CAD build for the part. Positions are in the model's coordinates, mm. Round coordinates to 2 decimals unless told otherwise and drop trailing zeros. Order: outer loops, then holes, each group sorted by start corner. A loop starts at its lowest first (then second) coordinate and runs counter-clockwise, first axis right, second up. Notation, with made-up numbers: M 49,-36 L 108,-36 A8 cw 108,-22 Z; hole C -10,-36.75 d1. An arc over 180 degrees is marked long. Answer as a JSON object with one key per item and string values.
```python
from build123d import *

# Parameters (mm, degrees)
F0_R     = 1.5875
F1_DEPTH = 3.048


# Not quite as in the source:
# - a feature names something its author has since deleted; it is built from what else it names


with BuildPart() as f1:
    # F0 (on Front) → F1 (new body)
    with BuildSketch(Plane.XZ):
        with BuildLine():
            Line((0, 3.0934604908), (0, 0))
            Line((0, 0), (0, -9.6065395092))
            ThreePointArc((0, -9.6065395092), (11.1386616751, -5.0428542466), (15.8731222627, 6.024299409))
            ThreePointArc((15.8731222627, 6.024299409), (15.8745305587, 6.1463763397), (15.875, 6.2684604908))
            ThreePointArc((15.875, 6.2684604908), (15.8438414904, 7.2625992274), (15.7504882737, 8.2528354908))
            ThreePointArc((15.7504882737, 8.2528354908), (10.5003255158, 18.1747104908), (0, 22.1434604908))
            Line((0, 22.1434604908), (0, 9.4434604908))
            ThreePointArc((0, 9.4434604908), (2.2450640303, 8.513524521), (3.175, 6.2684604908))
            ThreePointArc((3.175, 6.2684604908), (2.2450640303, 4.0233964605), (0, 3.0934604908))
        make_face()
        with BuildLine():
            Line((0, -9.6065395092), (0, 0))
            Line((0, 0), (0, 3.0934604908))
            ThreePointArc((0, 3.0934604908), (-3.175, 6.2684604908), (0, 9.4434604908))
            Line((0, 9.4434604908), (0, 22.1434604908))
            ThreePointArc((0, 22.1434604908), (-10.5003255158, 18.1747104908), (-15.7504882737, 8.2528354908))
            ThreePointArc((-15.7504882737, 8.2528354908), (-15.8510182356, 7.1407252981), (-15.8731222627, 6.024299409))
            ThreePointArc((-15.8731222627, 6.024299409), (-11.1386616751, -5.0428542466), (0, -9.6065395092))
        make_face()
        with BuildLine():
            ThreePointArc((15.8731222627, 6.024299409), (11.1386616751, -5.0428542466), (0, -9.6065395092))
            Line((0, -9.6065395092), (0, -42.3331838364))
            ThreePointArc((0, -42.3331838364), (10.5347283248, -46.6968111845), (14.8983556728, -57.2315395092))
            Line((14.8983556728, -57.2315395092), (36.5125, -57.2315395092))
            ThreePointArc((36.5125, -57.2315395092), (39.2955109449, -51.1953860295), (45.6930099416, -49.3919711196))
            Line((45.6930099416, -49.3919711196), (21.9056452954, -45.6203437456))
            ThreePointArc((21.9056452954, -45.6203437456), (17.0653083108, -42.8843212703), (15.2013844237, -37.6459561768))
            Line((15.2013844237, -37.6459561768), (15.8731222627, 6.024299409))
        make_face()
        with BuildLine():
            Line((0, -42.3331838364), (0, -9.6065395092))
            ThreePointArc((0, -9.6065395092), (-11.1386616751, -5.0428542466), (-15.8731222627, 6.024299409))
            Line((-15.8731222627, 6.024299409), (-14.8965934556, -57.4606795809))
            ThreePointArc((-14.8965934556, -57.4606795809), (-10.6154324462, -46.778138353), (0, -42.3331838364))
        make_face()
        with BuildLine():
            ThreePointArc((14.8983556728, -57.2315395092), (10.5347283248, -46.6968111845), (0, -42.3331838364))
            Line((0, -42.3331838364), (0, -54.0565395092))
            ThreePointArc((0, -54.0565395092), (2.2450640303, -54.986475479), (3.175, -57.2315395092))
            Line((3.175, -57.2315395092), (14.8983556728, -57.2315395092))
        make_face()
        with BuildLine():
            Line((0, -54.0565395092), (0, -42.3331838364))
            ThreePointArc((0, -42.3331838364), (-10.6154324462, -46.778138353), (-14.8965934556, -57.4606795809))
            ThreePointArc((-14.8965934556, -57.4606795809), (-9.5873458416, -68.6352144199), (2.3330776963, -71.9460816433))
            ThreePointArc((2.3330776963, -71.9460816433), (11.32960774, -66.9062999823), (14.8983556728, -57.2315395092))
            Line((14.8983556728, -57.2315395092), (3.175, -57.2315395092))
            ThreePointArc((3.175, -57.2315395092), (-2.2450640303, -59.4766035395), (0, -54.0565395092))
        make_face()
        with BuildLine():
            Line((36.5125, -57.2315395092), (14.8983556728, -57.2315395092))
            ThreePointArc((14.8983556728, -57.2315395092), (11.32960774, -66.9062999823), (2.3330776963, -71.9460816433))
            Line((2.3330776963, -71.9460816433), (45.6930099416, -65.0711078988))
            ThreePointArc((45.6930099416, -65.0711078988), (39.2955109449, -63.2676929889), (36.5125, -57.2315395092))
        make_face()
        with BuildLine():
            Line((-9.4502929642, 58.2590854908), (-15.7504882737, 8.2528354908))
            ThreePointArc((-15.7504882737, 8.2528354908), (-10.5003255158, 18.1747104908), (0, 22.1434604908))
            Line((0, 22.1434604908), (0, 44.3480842421))
            Line((0, 44.3480842421), (0, 47.5434604908))
            ThreePointArc((0, 47.5434604908), (-7.14375, 50.7682651813), (-9.4502929642, 58.2590854908))
        make_face()
        with Locations((-1.5875, 44.3480842421)):
            Circle(F0_R, mode=Mode.SUBTRACT)
        with BuildLine():
            Line((0, 44.3480842421), (0, 22.1434604908))
            ThreePointArc((0, 22.1434604908), (10.5003255158, 18.1747104908), (15.7504882737, 8.2528354908))
            Line((15.7504882737, 8.2528354908), (9.4502929642, 58.2590854908))
            ThreePointArc((9.4502929642, 58.2590854908), (9.5063048942, 57.6649437327), (9.525, 57.0684604908))
            ThreePointArc((9.525, 57.0684604908), (6.7351920908, 50.3332684), (0, 47.5434604908))
            Line((0, 47.5434604908), (0, 44.3480842421))
        make_face()
        with BuildLine():
            ThreePointArc((45.6930099416, -49.3919711196), (39.2955109449, -51.1953860295), (36.5125, -57.2315395092))
            ThreePointArc((36.5125, -57.2315395092), (39.2955109449, -63.2676929889), (45.6930099416, -65.0711078988))
            ThreePointArc((45.6930099416, -65.0711078988), (50.4861534797, -62.3860285644), (52.3875, -57.2315395092))
            ThreePointArc((52.3875, -57.2315395092), (50.4861534797, -52.0770504541), (45.6930099416, -49.3919711196))
        make_face()
        with BuildLine():
            ThreePointArc((47.625, -57.2315395092), (44.45, -60.4065395092), (41.275, -57.2315395092))
            ThreePointArc((41.275, -57.2315395092), (44.45, -54.0565395092), (47.625, -57.2315395092))
        make_face(mode=Mode.SUBTRACT)
        with BuildLine():
            ThreePointArc((9.4502929642, 58.2590854908), (0, 66.5934604908), (-9.4502929642, 58.2590854908))
            ThreePointArc((-9.4502929642, 58.2590854908), (-7.14375, 50.7682651813), (0, 47.5434604908))
            ThreePointArc((0, 47.5434604908), (6.7351920908, 50.3332684), (9.525, 57.0684604908))
            ThreePointArc((9.525, 57.0684604908), (9.5063048942, 57.6649437327), (9.4502929642, 58.2590854908))
        make_face()
        with BuildLine():
            ThreePointArc((3.175, 57.0684604908), (2.2450640303, 54.8233964605), (0, 53.8934604908))
            ThreePointArc((0, 53.8934604908), (-2.2450640303, 59.313524521), (3.175, 57.0684604908))
        make_face(mode=Mode.SUBTRACT)
    extrude(amount=F1_DEPTH)


solid = f1.part
```
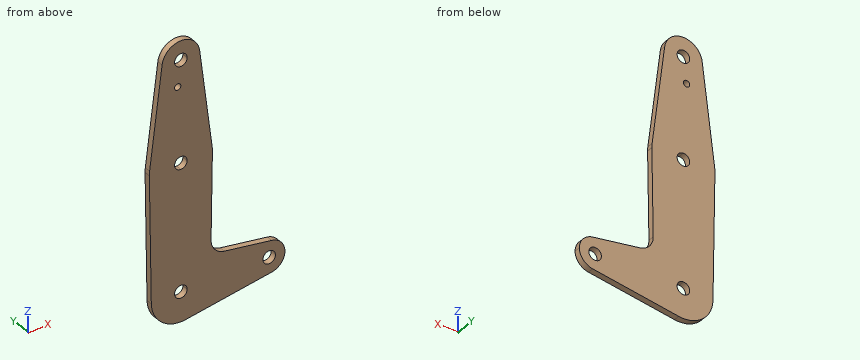
Item 1: Saw through at C-C on z = -11.5. List the corners of the cut face in (x, y).
Worked answers:
{"outline": "M -15.6,-3.05 L 15.6,-3.05 L 15.6,0 L -15.6,0 Z"}
Item 2: Saw through at D-D on x = 13. List the corners of the cut face in (y, z).
Worked answers:
{"outline": "M -3.05,-70.25 L 0,-70.25 L 0,30.08 L -3.05,30.08 Z"}
Item 3: Saw through at A-A on x = 44.45. List the corners of the cut face in (y, z), and give its area (3 significant figures).
Worked answers:
{"outline": "M -3.05,-65.27 L 0,-65.27 L 0,-60.41 L -3.05,-60.41 Z; M -3.05,-54.06 L 0,-54.06 L 0,-49.19 L -3.05,-49.19 Z", "area": "29.6 mm2"}
Item 4: Wall check: line 1 along X through (y, z) = (-0.8, -57); line 2 along Z through (x, y) = (-1.5, -2.8); line 3 along X through (y, z) = (-0.5, -1). Give the ranges that are in metal, low to high. Write a range as [from, to].
Worked answers:
{"line 1": "x = [-14.9, -3.17], [3.17, 41.28], [47.62, 52.38]", "line 2": "z = [-72.05, -60.03], [-54.43, 3.47], [9.07, 42.76], [45.93, 54.27], [59.87, 66.47]", "line 3": "x = [-15.77, 15.77]"}
Item 5: Saw through at B-B on y = -1. State how many separate pieces and enclosed holes the cut face has, and give its area (3 significant figures).
Worked answers:
{"separate pieces": "1", "enclosed holes": "5", "area": "4,360 mm2"}
Item 6: Drop flat-ended pins along their axis: pin 1 Ø1.5 at (x, y) = (45.5, -2.5) entering from -Z; pin 2 Ø3 at (x, z) = (-1.59, 44.35) entering from +Y; pin 3 Ø1 at (y, z) = (-2.5, -57.5) entering from -X; pin 4 Ø8.5 at (x, z) = (0, 57.07) entering from +Y. Give the stop position or say it passes through.
Worked answers:
{"pin 1": "stops at z = -65.22", "pin 2": "passes through", "pin 3": "stops at x = -14.9", "pin 4": "stops at y = 0"}
